```python
from build123d import *

# Parameters (mm, degrees)
F0_W     = 9.525
F0_H     = 4.572
F1_DEPTH = 25.4
F2_R     = 2.2225
F3_DEPTH = 10.923
F4_R     = 4.0386
F5_DEPTH = 5.08


with BuildPart() as f1:
    # F0 (on Front) → F1 (new body)
    with BuildSketch(Plane.XZ):
        with Locations((4.7625, 2.286)):
            Rectangle(F0_W, F0_H)
        Polygon((9.525, 0), (0, 0), (-1.2375, 0), (-1.2375, -6.35), (10.7625, -6.35), (10.7625, 0), align=None)
    extrude(amount=F1_DEPTH)

    # F2 (on face) → F3 (cut, through all)
    with BuildSketch(Plane.XY.offset(4.572)):
        with Locations((4.7625, -12.7)):
            Circle(F2_R)
    extrude(amount=-F3_DEPTH, mode=Mode.SUBTRACT)

    # F4 (on face) → F5 (cut)
    with BuildSketch(Plane(origin=(0, 0, -6.35), x_dir=(1, 0, 0), z_dir=(0, 0, -1))):
        with Locations((4.7625, 12.7)):
            Circle(F4_R)
    extrude(amount=-F5_DEPTH, mode=Mode.SUBTRACT)


solid = f1.part
```
Can you work these out from the model? Positions are in its coordinate system, mm. A direction names the side the tool comes from. Give positions to 0.01 mm unless a question says otherwise; leave off trailing zeros. Loops run counter-clockwise (first coordinate to the right, second up) from the corner with the lowest first, then second, coordinate; pieces in that order, holes last. Notation, with made-up numbers: M -3,-25.5 L 49,-25.5 A16 ccw 49,-18.5 Z; hole C 77,1.25 d5. An arc over 180 degrees is marked long. One line per question, with ' | ' between items. Start each with the question number.
Q1. For pin 1 Ø0.6 at (x, y) = (10, -15) entering from +Z; pin 2 Ø1.4 at (y, z) = (-16.5, 2.5) entering from -X; pin 3 Ø2.5 at (x, y) = (4.76, -12.7) entering from -Z, each with a flat end and sliding along its axis, tell me the tip position at first contact or that it passes through.
Q2. If we mould it in two halves opening along X, with no side actions, what happens to faces 1 (the flat face through (5, 0, -1)), 2 (the cylindrical face through (1.56, -10.24, -3.85)), 3 (the flat face through (10.762, -13, -3))? For each: +X half, -X half, draft (parallel to the pull), parting line (faces both ways), or undercut.
Q3. For faces 4 (the flat face through (7, -11, -1.27)), 5 (the flat face through (9.525, -13, 2)), 6 (the flat face through (1, -10, -6.35)), 7 (the flat face through (0, -13, 2)), 8 (the flat face through (4.7, -15.3, 4.572)), which set-ups out of +Z, -Z, +X, -X, +Y, -Y let a thin tool reach every point of the face, with its end or its side?
Q4. If we section it at C-C (z = 2.25): Please give me the cut outline in (x, y) (1 decimal).
Q5. If I drill on line 1 (X direction, y = -12.7, z = -4.5); line 2 (Y direction, x = 4.75, z = -2.75); line 3 (X direction, y = -1.5, z = 3) (3 decimals), over which ranges is the centre line in solid material (lowest first)? Write a range as from..to.
Q6. If we section it at B-B (x = 3.75): Please give me the cut outline in (y, z), plus the area to 3 significant figures.
Computed:
1) pin 1: stops at z = 0 | pin 2: stops at x = 0 | pin 3: passes through
2) face 1: draft | face 2: undercut | face 3: +X half
3) face 4: -Z | face 5: +Z, +X, +Y, -Y | face 6: -Z, +X, -X, +Y, -Y | face 7: +Z, -X, +Y, -Y | face 8: +Z, +X, -X, +Y, -Y
4) outline: M 0,-25.4 L 9.5,-25.4 L 9.5,0 L 0,0 Z; hole C 4.8,-12.7 d4.4
5) line 1: x = -1.24..0.72, 8.8..10.76 | line 2: y = -25.4..-16.74, -8.66..0 | line 3: x = 0..9.525
6) outline: M -25.4,-6.35 L -16.61,-6.35 L -16.61,-1.27 L -14.68,-1.27 L -14.68,4.57 L -25.4,4.57 Z; M -10.72,-1.27 L -8.79,-1.27 L -8.79,-6.35 L 0,-6.35 L 0,4.57 L -10.72,4.57 Z | area: 215 mm²
